```python
from build123d import *

# Parameters (mm, degrees)
BOSS_EXTRUDE1_DEPTH     = 5
CUT_EXTRUDE8_DEPTH      = 10.848857802
CUT_EXTRUDE8_DEPTH_BACK = 10.848857802
REVOLVE1_ANGLE          = 180
SKETCH24_W              = 3.9
SKETCH24_H              = 6
BOSS_EXTRUDE2_DEPTH     = 4
SKETCH25_W              = 3.9
SKETCH25_H              = 3
REVOLVE2_ANGLE          = 180
SKETCH26_R              = 1.45
CUT_EXTRUDE9_DEPTH      = 19
BOSS_EXTRUDE4_DEPTH     = 3.7


with BuildPart() as part:
    # Sketch2 → Boss-Extrude1 (new, symmetric)
    with BuildSketch(Plane(origin=(0, 0, 0), x_dir=(1, 0, 0), z_dir=(0, 1, 0))):
        Polygon((-3, 6), (3, 6), (6, 3), (6, -3), (3, -6), (-3, -6), (-6, -3), (-6, 3), align=None)
    extrude(amount=BOSS_EXTRUDE1_DEPTH, both=True)

    # Sketch22 → Cut-Extrude8 (cut, two sides: drawn at the far end of the back side and taken through both)
    with BuildSketch(Plane(origin=(0, 0, 0), x_dir=(0, 0, -1), z_dir=(1, 0, 0)).offset(-CUT_EXTRUDE8_DEPTH_BACK)):
        Polygon((0, -5), (-6, -5), (-6, -1.535898385), align=None)
    extrude(amount=CUT_EXTRUDE8_DEPTH + CUT_EXTRUDE8_DEPTH_BACK, mode=Mode.SUBTRACT)

    # Sketch23 → Revolve1 (revolve)
    with BuildSketch(Plane(origin=(0, 5, 0), x_dir=(1, 0, 0), z_dir=(0, 1, 0))):
        Polygon((-6, 0), (-6, 3), (-3, 6), (3, 6), (6, 3), (6, 0), align=None)
    revolve(axis=Axis((6, 5, 0), (1, 0, 0)), revolution_arc=REVOLVE1_ANGLE)

    # Sketch24 → Boss-Extrude2 (add, symmetric)
    with BuildSketch(Plane.XZ.offset(5)):
        with Locations((-4.05, 0)):
            Rectangle(SKETCH24_W, SKETCH24_H)
    boss_extrude2 = extrude(amount=BOSS_EXTRUDE2_DEPTH, both=True)

    # Sketch25 → Revolve2 (revolve)
    with BuildSketch(Plane.XZ.offset(9)):
        with Locations((-4.05, 1.5)):
            Rectangle(SKETCH25_W, SKETCH25_H)
    revolve2 = revolve(axis=Axis((-6, -9, 0), (1, 0, 0)), revolution_arc=REVOLVE2_ANGLE)

    # Sketch26 → Cut-Extrude9 (cut, symmetric)
    with BuildSketch(Plane.ZY.offset(6)):
        with Locations((0, -9)):
            Circle(SKETCH26_R)
    cut_extrude9 = extrude(amount=CUT_EXTRUDE9_DEPTH, both=True, mode=Mode.SUBTRACT)

    # Mirror1: Boss-Extrude2, Revolve2, Cut-Extrude9 across plane
    add(boss_extrude2.mirror(Plane(origin=(0, 0, 0), x_dir=(0, 0, 1), z_dir=(1, 0, 0))))
    add(revolve2.mirror(Plane(origin=(0, 0, 0), x_dir=(0, 0, 1), z_dir=(1, 0, 0))))
    add(cut_extrude9.mirror(Plane(origin=(0, 0, 0), x_dir=(0, 0, 1), z_dir=(1, 0, 0))), mode=Mode.SUBTRACT)

    # Sketch30 → Cut-Revolve1 (revolve, cut)
    with BuildSketch(Plane(origin=(0, -3.75, 2.165063509), x_dir=(1, 0, 0), z_dir=(0, -0.8660254037844418, 0.49999999999999484))):
        Polygon((0, 3.42820323), (-0.75, 2.67820323), (-0.75, 1.92820323), (0.75, 1.92820323), (0.75, 2.67820323), align=None)
    revolve(axis=Axis((-6, -1.535898385, 6), (1, 0, 0)), mode=Mode.SUBTRACT)

    # Sketch34 → Boss-Extrude4 (add)
    with BuildSketch(Plane.XZ.offset(5)):
        Polygon((-6, -3), (-2.1, -3), (2.1, -3), (6, -3), (3, -6), (-3, -6), align=None)
    extrude(amount=BOSS_EXTRUDE4_DEPTH)

    # Sketch35 → Cut-Revolve3 (revolve, cut)
    with BuildSketch(Plane.XZ.offset(8.7)):
        Polygon((0, -3.5), (-0.75, -4.25), (-0.75, -5), (0.75, -5), (0.75, -4.25), align=None)
    revolve(axis=Axis((3, -8.7, -6), (1, 0, 0)), mode=Mode.SUBTRACT)


solid = part.part
```
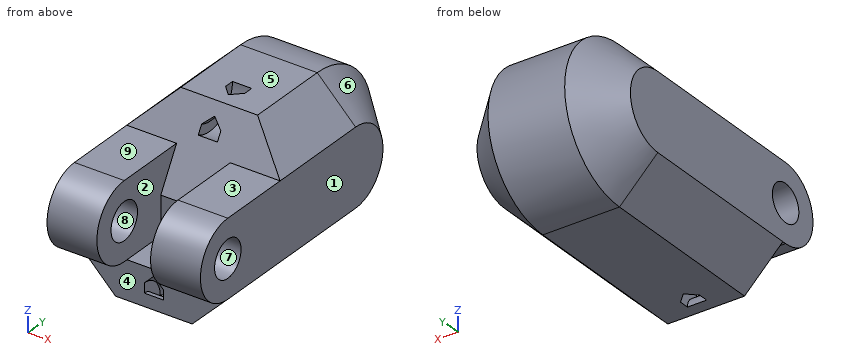
Could you check a few things on this model? Use its own coordinates, in mm. Face numbers are marked on the shaded views. A direction names the side the tool comes from. Coordinates: 2 decimals unless noted, no trailing zeros. Order: outer loops, then holes, each group sorted by start corner. A loop starts at its lowest first (then second) coordinate and runs counter-clockwise, first axis right, second up. Notation, with made-up numbers: M 63.25,85.5 L 108.25,85.5 A27 ccw 108.25,123.5 Z; hole C -39.75,45 d7. An arc over 180 degrees is marked long. Use one line per item in the form item = value. Start each with the question number.
1. Please list where these lines run through material, in increasing order: line 1 (Z direction, x = 4.7, y = -9); line 2 (X direction, y = -10.5, z = 2.25); line 3 (Y direction, x = 3.2, z = 0).
2. Suppose I cut it at A-A on x = -1.75. Write out the boundary of the cut face in (y, z).
3. We'd pull the mould along Y, two halves only. Please class the marked faces 6, 7, 8 and 9: +Y half, -Y half, draft (parallel to the pull), parting line (faces both ways), or undercut.
4. Suppose I cut it at B-B on x = 4.25. Write out the boundary of the cut face in (y, z), then the cut area to 3 significant figures.
5. Suppose I cut it at C-C on y = -8. Count the separate pieces of the cut face and the enclosed holes in it, then the cut area to 3 significant figures.
6. On a 3-axis mill with a long thin cutter (end or side, diameter ignored), from which of +Z, -Z, +X, -X, +Y, -Y can I reach the whole of each face in a straight line? I mean the marked faces 1, 2, 3, 4 and 5. Say none if no direction works.
7. For pin 1 (3.5 mm diameter, centred on x = 0, z = -2, fed in from -Y); pin 2 (2 mm diameter, centred on x = 4.5, y = 7.5, fed in from +Z); pin 3 (3 mm diameter, centred on x = 0.5, y = -7.5, fed in from +Z), each with a flat end and sliding along its axis, tell me the tip position at first contact or that it passes through.
Geometry says:
q1.line_1 = -3 to -1.45, 1.45 to 3
q1.line_2 = -6 to -2.1, 2.1 to 6
q1.line_3 = -12 to -10.45, -7.55 to 10.8
q2.outline = M -8.7,-6 L 5,-6 A6 ccw 5,6 L -1.54,6 L -5,0 L -5,-3 L -8.7,-3 Z
q3.face_6 = +Y half
q3.face_7 = undercut
q3.face_8 = undercut
q3.face_9 = draft
q4.outline = M -9,-3 L -8.7,-3 L -8.7,-4.75 L 5,-4.75 A4.75 ccw 5,4.75 L -2.26,4.75 L -3.27,3 L -9,3 A3 ccw Z; hole C -9,0 d2.9
q4.area = 165 mm^2
q5.separate_pieces = 3
q5.enclosed_holes = 1
q5.area = 55.5 mm^2
q6.face_1 = +Z, -Z, +X, +Y, -Y
q6.face_2 = +Z, -Y
q6.face_3 = +Z, +X, -X, -Y
q6.face_4 = -Z, +X, -X, -Y
q6.face_5 = +Z, +X, -X, +Y, -Y
q7.pin_1 = -8.7
q7.pin_2 = 4.99
q7.pin_3 = -3
